Work out the finished part from the listing and answer in its coordinate system (mm). A direction names the side the tool comes from. Round coordinates to 2 decimals unless told otherwise and drop trailing zeros. Loops run counter-clockwise (first coordinate to the right, second up) from the corner with the lowest first, then second, coordinate; pieces in that order, holes last. Notation, with made-up numbers: (65, -0.5) -> (80, -0.5) arc R29 ccw to (80, 38.5) -> close; hole circle Ø8 at (-38.5, 15). An arc over 180 degrees is marked (long way). Use CSV: the item, a comma, the result in double quotes. Start each with the question number.
from build123d import *

# Parameters (mm, degrees)
PAD_DEPTH       = 29.5
POCKET_DEPTH    = 19.5
POCKET001_DEPTH = 6.9
POCKET002_DEPTH = 5
POCKET003_DEPTH = 5
SKETCH006_R     = 9.5
POCKET004_DEPTH = 56
POCKET005_DEPTH = 100


with BuildPart() as part:
    # Sketch → Pad (new body)
    with BuildSketch(Plane.XY):
        Polygon((-31.5, 98.35), (-31.5, 45.1), (-21, 25.1), (-21, -28.9), (14, -28.9), (14, -22), (21, -22), (21, 25.2), (31.5, 45.1), (31.5, 98.35), (26.5, 98.35), (26.5, 50.1), (-26.5, 50.1), (-26.5, 98.35), align=None)
        Polygon((-18.875, 40.1), (-11, 25.1), (-5, 25.1), (-5, 40.1), align=None, mode=Mode.SUBTRACT)
        Polygon((5, 40.1), (5, 25.2), (11, 25.2), (18.861809, 40.1), align=None, mode=Mode.SUBTRACT)
    extrude(amount=PAD_DEPTH)

    # Sketch001 → Pocket (cut)
    with BuildSketch(Plane.XY.offset(5)):
        Polygon((-15.5, 18.3), (-15.5, -22), (11.5, -22), (11.5, -28.9), (14, -28.9), (14, -22), (21, -22), (21, -18), (27.5, -18), (27.5, -12), (21, -12), (21, 12.3), (21, 12.3), (21, 18.3), (21, 18.3), (21, 25.15), (11.5, 25.15), (11.5, 18.3), align=None)
    extrude(amount=POCKET_DEPTH, mode=Mode.SUBTRACT)

    # Sketch003 → Pocket001 (cut)
    with BuildSketch(Plane(origin=(-15.5, -28.9, 5), x_dir=(1, 0, 0), z_dir=(0, -1, 0))):
        Polygon((20.030856, 9.535838), (10, 0), (0, 0), (0, 19.5), (20, 19.5), align=None)
    extrude(amount=-POCKET001_DEPTH, mode=Mode.SUBTRACT)

    # Sketch004 → Pocket002 (cut)
    with BuildSketch(Plane.XY.offset(5)):
        Polygon((-16, 18.3), (-16, -17), (9, -17), (9, -16.114332), (9, 18.3), align=None)
    extrude(amount=-POCKET002_DEPTH, mode=Mode.SUBTRACT)

    # Sketch005 → Pocket003 (cut)
    with BuildSketch(Plane.XY.offset(29.5)):
        Polygon((-16, 18.3), (-16, -22), (7, -22), (7, -16.175392), (16, -16.175392), (16, 18.3), align=None)
    extrude(amount=-POCKET003_DEPTH, mode=Mode.SUBTRACT)

    # Sketch006 → Pocket004 (cut)
    with BuildSketch(Plane(origin=(-22, -27.65, 3), x_dir=(0, 1, 0), z_dir=(1, 0, 0))):
        with Locations((16.005131, 11.909992)):
            Circle(SKETCH006_R)
    extrude(amount=POCKET004_DEPTH, mode=Mode.SUBTRACT)

    # Sketch007 → Pocket005 (cut)
    with BuildSketch(Plane(origin=(-50, 83.6, 14.75), x_dir=(0, 1, 0), z_dir=(1, 0, 0))):
        with BuildLine():
            ThreePointArc((4.2e-05, -14.75), (14.75, 3.4e-05), (-2.6e-05, 14.75))
            Line((-2.6e-05, 14.75), (14.750042, 14.750026))
            Line((14.750042, 14.750026), (14.750042, -14.75))
            Line((14.750042, -14.75), (4.2e-05, -14.75))
        make_face()
    extrude(amount=POCKET005_DEPTH, mode=Mode.SUBTRACT)


solid = part.part
Q1. Section A-A, the plane z = 17 is taken. Give the number of separate pieces and of enclosed holes in the cut face, and give its area (3 significant figures).
Q2. Section D-D, the plane y = 85 is taken. Write down the section's boundary in (x, z).
Q3. Section B-B, the plane y = 62 is taken. Write down the section's boundary in (x, z), and give its area (3 significant figures).
Q4. Each of these flat-tipped pins is pushed along its axis until it touches: pin 1 (4 mm diameter, centred on y = -26, z = 26.5, fed in from +X); pin 2 (4 mm diameter, centred on x = 16.5, z = 27, fed in from -Y); pin 3 (1 mm diameter, centred on x = 6.5, z = 24, fed in from +Y); pin 4 (6 mm diameter, centred on x = -7.5, y = 12.5, fed in from +Z). Where does it stop, or does it pass through?
Q5. Which of the six approach directions +Z, -Z, +X, -X, +Y, -Y give full straight-line access (tool end or side, diameter ignored) to faces 5 (the flat face through (7, -22, 20)), 6 (the flat face through (0, 50.1, 15)), 7 (the flat face through (17, -22, 27))?
Q6. Section C-C, the plane y = 7 is taken. Write down the section's boundary in (x, z), and give its area (3 significant figures).
Q7. Straight lines are drawn through the part: line 1 (X direction, y = 66.5, z = 12.75); line 2 (X direction, y = 29.5, z = 22); line 3 (X direction, y = -3.5, z = 4.5). For each, find the intervals that lie inside material, in ascending order. Write a range as from..to.
Q8. For a pull along Y with two mould halves and no side action, classify faces 1 (the flat face through (31.5, 71, 15)), 2 (the flat face through (16, 1, 27)), 3 (the flat face through (-26.324, 35.24, 14.544)), 4 (the cylindrical face through (28.965, 98.346, 14.426)) as pulls with the +Y half, pulls with the -Y half, needs draft (parallel to the pull), parting line crosses it, or undercut.
Report:
1,separate pieces,"3"
1,enclosed holes,"2"
1,area,"1,970 mm²"
2,outline,"(-31.5, 0.07) -> (-26.5, 0.07) -> (-26.5, 29.43) -> (-31.5, 29.43) -> close; (26.5, 0.07) -> (31.5, 0.07) -> (31.5, 29.43) -> (26.5, 29.43) -> close"
3,outline,"(-31.5, 0) -> (-26.5, 0) -> (-26.5, 29.5) -> (-31.5, 29.5) -> close; (26.5, 0) -> (31.5, 0) -> (31.5, 29.5) -> (26.5, 29.5) -> close"
3,area,"295 mm²"
4,pin 1,"stops at x = 14"
4,pin 2,"stops at y = -22"
4,pin 3,"stops at y = 50.1"
4,pin 4,"passes through"
5,face 5,"none"
5,face 6,"+Z, -Z, +Y"
5,face 7,"+Z, -Z, +X, -Y"
6,outline,"(-21, 0) -> (-16, 0) -> (-16, 5) -> (-15.5, 5) -> (-15.5, 24.5) -> (-16, 24.5) -> (-16, 29.5) -> (-21, 29.5) -> close; (9, 0) -> (21, 0) -> (21, 5) -> (9, 5) -> close; (16, 24.5) -> (21, 24.5) -> (21, 29.5) -> (16, 29.5) -> close"
6,area,"242 mm²"
7,line 1,"x = -31.5..-26.5, 26.5..31.5"
7,line 2,"x = -23.31..-13.31, -5..5, 13.27..23.27"
7,line 3,"x = -21..-16, 9..21"
8,face 1,"needs draft"
8,face 2,"undercut"
8,face 3,"pulls with the -Y half"
8,face 4,"pulls with the +Y half"
